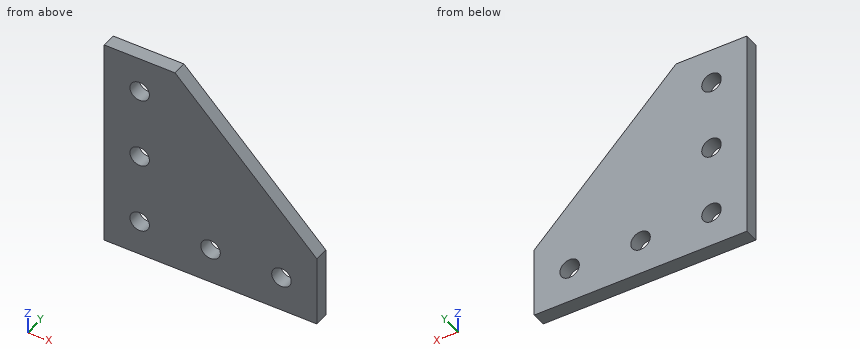
```python
from build123d import *

# Parameters (mm, degrees)
F0_R     = 2.75
F1_DEPTH = 4


with BuildPart() as f1:
    # F0 (on Front) → F1 (new body)
    with BuildSketch(Plane.XZ):
        Polygon((-15.552693, 34.197687), (-35.552693, 34.197687), (-35.552693, -25.802313), (24.447307, -25.802313), (24.447307, -5.802313), align=None)
        with Locations((-25.552693, -15.802313)):
            Circle(F0_R, mode=Mode.SUBTRACT)
        with Locations((-5.552693, -15.802313)):
            Circle(F0_R, mode=Mode.SUBTRACT)
        with Locations((-25.552693, 4.197687)):
            Circle(F0_R, mode=Mode.SUBTRACT)
        with Locations((14.447307, -15.802313)):
            Circle(F0_R, mode=Mode.SUBTRACT)
        with Locations((-25.552693, 24.197687)):
            Circle(F0_R, mode=Mode.SUBTRACT)
    extrude(amount=F1_DEPTH)


solid = f1.part
```
Design review of the part built by this model. Coordinates are the model's own, in mm. Coordinates: 2 decimals unless noted, no trailing zeros. Order: outer loops, then holes, each group sorted by start corner. A loop starts at its lowest first (then second) coordinate and runs counter-clockwise, first axis right, second up. Notation, with made-up numbers: (22, 52) - (50, 52) arc R22 ccw to (50, 79) - close; hole circle Ø3 at (13, 86). An arc over 180 degrees is marked (long way). Answer in a Markdown table with one row per item.
(1) Consider section C-C on z = -1. State the section outline as (x, y) points (3 decimals), plus the area to 3 significant figures.
Checked values:
| item | result |
|---|---|
| outline | (-35.553, -4) - (19.645, -4) - (19.645, 0) - (-35.553, 0) - close |
| area | 221 mm^2 |
(2) Consider section D-D on x = 2. State the section outline as (y, z) points (3 decimals).
Checked values:
| item | result |
|---|---|
| outline | (-4, -25.802) - (0, -25.802) - (0, 16.645) - (-4, 16.645) - close |
(3) Consider section A-A on x = 15.5. State the section outline as (y, z) points (3 decimals), plus the area to 3 significant figures.
Checked values:
| item | result |
|---|---|
| outline | (-4, -25.802) - (0, -25.802) - (0, -18.343) - (-4, -18.343) - close; (-4, -13.262) - (0, -13.262) - (0, 3.145) - (-4, 3.145) - close |
| area | 95.5 mm^2 |
(4) Consider section B-B on y = -2.5. State the section outline as (x, z) points, plus the area to 3 significant figures.
Checked values:
| item | result |
|---|---|
| outline | (-35.55, -25.8) - (24.45, -25.8) - (24.45, -5.8) - (-15.55, 34.2) - (-35.55, 34.2) - close; hole circle Ø5.5 at (-25.55, -15.8); hole circle Ø5.5 at (-25.55, 4.2); hole circle Ø5.5 at (-25.55, 24.2); hole circle Ø5.5 at (-5.55, -15.8); hole circle Ø5.5 at (14.45, -15.8) |
| area | 2,680 mm^2 |
(5) Wall thickness on line 1 along Z through (x, y) = (15, -2.6) (3 decimals); line 2 along X through (y, z) = (-1.8, 4.5) (3 decimals); line 3 along X through (y, z) = (-1.15, 14.5) (3 decimals): over which ranges is each line inside the solid? List them lowest first. Write a range as from..to.
Checked values:
| item | result |
|---|---|
| line 1 | -25.802..-18.496, -13.108..3.645 |
| line 2 | -35.553..-28.286, -22.819..14.145 |
| line 3 | -35.553..4.145 |
(6) Clearance check with flat-ended pins moving along their axes: pin 1 (7 mm diameter, centred on x = -25.55, z = 4.2, fed in from +Y); pin 2 (1 mm diameter, centred on x = 17.5, y = -2.5, fed in from +Z) (3 decimals); pin 3 (4.5 mm diameter, centred on x = -5.55, z = -15.8, fed in from -Y). State where each tip first meets the part, or that it passes through.
Checked values:
| item | result |
|---|---|
| pin 1 | y = 0 |
| pin 2 | z = 1.645 |
| pin 3 | through |
